from build123d import *

# Parameters (mm, degrees)
BOSS_EXTRUDE1_DEPTH = 2
SKETCH2_R           = 3.5
SKETCH2_R_2         = 2.5
BOSS_EXTRUDE2_DEPTH = 6
SKETCH3_R           = 1.25
CUT_EXTRUDE1_DEPTH  = 1
SKETCH4_R           = 0.5
CUT_EXTRUDE2_DEPTH  = 1


with BuildPart() as part:
    # Sketch1 → Boss-Extrude1 (new body)
    with BuildSketch(Plane.XY):
        with BuildLine():
            Line((1.653818246, -7.701405378), (2.100322305, -3.726408024))
            ThreePointArc((2.100322305, -3.726408024), (2.127371286, -3.184526841), (2.395247592, -2.712712102))
            ThreePointArc((2.395247592, -2.712712102), (2.55393801, -2.55393801), (2.712712102, -2.395247592))
            ThreePointArc((2.712712102, -2.395247592), (3.184526841, -2.127371286), (3.726408024, -2.100322305))
            Line((3.726408024, -2.100322305), (7.701405378, -1.653818246))
            ThreePointArc((7.701405378, -1.653818246), (8.713646486, -1.093206236), (9.092879943, 0))
            ThreePointArc((9.092879943, 0), (8.713646486, 1.093206236), (7.701405378, 1.653818246))
            Line((7.701405378, 1.653818246), (3.726408024, 2.100322305))
            ThreePointArc((3.726408024, 2.100322305), (3.184526841, 2.127371286), (2.712712102, 2.395247592))
            ThreePointArc((2.712712102, 2.395247592), (2.537508652, 2.537508652), (2.395247592, 2.712712102))
            ThreePointArc((2.395247592, 2.712712102), (2.127371286, 3.184526841), (2.100322305, 3.726408024))
            Line((2.100322305, 3.726408024), (1.653818246, 7.701405378))
            ThreePointArc((1.653818246, 7.701405378), (1.093206236, 8.713646486), (0, 9.092879943))
            ThreePointArc((0, 9.092879943), (-1.093206236, 8.713646486), (-1.653818246, 7.701405378))
            Line((-1.653818246, 7.701405378), (-2.100322305, 3.726408024))
            ThreePointArc((-2.100322305, 3.726408024), (-2.127371286, 3.184526841), (-2.395247592, 2.712712102))
            ThreePointArc((-2.395247592, 2.712712102), (-2.537508652, 2.537508652), (-2.712712102, 2.395247592))
            ThreePointArc((-2.712712102, 2.395247592), (-3.184526841, 2.127371286), (-3.726408024, 2.100322305))
            Line((-3.726408024, 2.100322305), (-7.701405378, 1.653818246))
            ThreePointArc((-7.701405378, 1.653818246), (-8.713646486, 1.093206236), (-9.092879943, 0))
            ThreePointArc((-9.092879943, 0), (-8.713646486, -1.093206236), (-7.701405378, -1.653818246))
            Line((-7.701405378, -1.653818246), (-3.726408024, -2.100322305))
            ThreePointArc((-3.726408024, -2.100322305), (-3.184526841, -2.127371286), (-2.712712102, -2.395247592))
            ThreePointArc((-2.712712102, -2.395247592), (-2.542453575, -2.542453575), (-2.395247592, -2.712712102))
            ThreePointArc((-2.395247592, -2.712712102), (-2.127371286, -3.184526841), (-2.100322305, -3.726408024))
            Line((-2.100322305, -3.726408024), (-1.653818246, -7.701405378))
            ThreePointArc((-1.653818246, -7.701405378), (-1.093206236, -8.713646486), (0, -9.092879943))
            ThreePointArc((0, -9.092879943), (1.093206236, -8.713646486), (1.653818246, -7.701405378))
        make_face()
    extrude(amount=BOSS_EXTRUDE1_DEPTH)

    # Sketch2 → Boss-Extrude2 (add)
    with BuildSketch(Plane(origin=(0, 0, 0), x_dir=(-1, 0, 0), z_dir=(0, 0, -1))):
        Circle(SKETCH2_R)
        Circle(SKETCH2_R_2, mode=Mode.SUBTRACT)
    extrude(amount=BOSS_EXTRUDE2_DEPTH)

    # Sketch3 → Cut-Extrude1 (cut)
    with BuildSketch(Plane.XY.offset(2)):
        Circle(SKETCH3_R)
    extrude(amount=-CUT_EXTRUDE1_DEPTH, mode=Mode.SUBTRACT)

    # Sketch4 → Cut-Extrude2 (cut)
    with BuildSketch(Plane.XY.offset(1)):
        Circle(SKETCH4_R)
    extrude(amount=-CUT_EXTRUDE2_DEPTH, mode=Mode.SUBTRACT)


solid = part.part
CAD build for the part. Positions are in the model's coordinates, mm. A direction names the side the tool comes from. Coordinates: 2 decimals unless noted, no trailing zeros. Write each loop counter-clockwise with the first axis right and the second up, starting at its lowest first coordinate (ties: lowest second). Pieces come first, ordered by that corner, then holes. Notation, with made-up numbers: M 45.25,-10 L 59.25,-10 A15 cw 59.25,16 Z; hole C -15,86 d3. An arc over 180 degrees is marked long. Return JSON: item names as keys, results as strings.
Item 1: Which spindle directions (+Z, -Z, +X, -X, +Y, -Y) get a long thin tool onto all of the face, cutting with end or side? Do faces 5 (the cylindrical face through (-3.233, -1.341, -2.958)), 6 (the flat face through (-1.874, 5.742, 0.986)), 7 (the flat face through (0, -1, 1)). Say none if no direction does.
Findings below:
{"face 5": "-Z", "face 6": "+Z, -Z, -X, +Y", "face 7": "+Z"}
Item 2: Slice it at A-A, the plane y = -0.25. Write the cut outline in (x, z).
Findings below:
{"outline": "M -9.08,0 L -3.49,0 L -3.49,-6 L -2.49,-6 L -2.49,0 L -0.43,0 L -0.43,1 L -1.22,1 L -1.22,2 L -9.08,2 Z; M 0.43,0 L 2.49,0 L 2.49,-6 L 3.49,-6 L 3.49,0 L 9.08,0 L 9.08,2 L 1.22,2 L 1.22,1 L 0.43,1 Z"}
Item 3: Slice it at D-D, the plane y = -4.5. Write the cut outline in (x, z), and give its area (3 significant figures).
Findings below:
{"outline": "M -2.01,0 L 2.01,0 L 2.01,2 L -2.01,2 Z", "area": "8.05 mm2"}
Item 4: Slice it at B-B, the plane z = -0.75. Write the cut outline in (x, y), and give its area (3 significant figures).
Findings below:
{"outline": "C 0,0 d7; hole C 0,0 d5", "area": "18.8 mm2"}
Item 5: Probe line 1 (X direction, y = -2, z = -4.5); line 2 (Y direction, x = -0.5, z = -4.25); line 3 (Z direction, x = 1.75, y = -6). List the from-to ranges inside material, lowest first. Write a range as from..to.
Findings below:
{"line 1": "x = -2.87..-1.5, 1.5..2.87", "line 2": "y = -3.46..-2.45, 2.45..3.46", "line 3": "z = 0..2"}
Item 6: Two-plate mould, pull along Y, no slides. Class faces 1 (the flat face through (-2, -2, -6)), 2 (the cylindrical face through (0.54, -2.44, -2.96)), 3 (the cylindrical face through (3.192, 2.125, 0.986)), 4 (the cylindrical face through (-0.27, -1.22, 1.51)): +Y half, -Y half, draft (parallel to the pull), parting line (faces both ways), or undercut.
Findings below:
{"face 1": "draft", "face 2": "undercut", "face 3": "+Y half", "face 4": "undercut"}
Item 7: Drop flat-ended pins along their axis: pin 1 Ø2 at (x, y) = (0, 0) entering from -Z; pin 2 Ø2 at (x, y) = (-2.5, -3) entering from +Z; pin 3 Ø1.5 at (x, z) = (7, -0.5) entering from -Y; pin 4 Ø4 at (x, z) = (0.5, -4) entering from -Y. Give the stop position or say it passes through.
Findings below:
{"pin 1": "stops at z = 0", "pin 2": "stops at z = 2", "pin 3": "stops at y = -1.8", "pin 4": "stops at y = -3.5"}
Item 8: Slice it at C-C, the plane x = 4.75. Write the cut outline in (y, z), and give its area (3 significant figures).
Findings below:
{"outline": "M -1.99,0 L 1.99,0 L 1.99,2 L -1.99,2 Z", "area": "7.94 mm2"}
